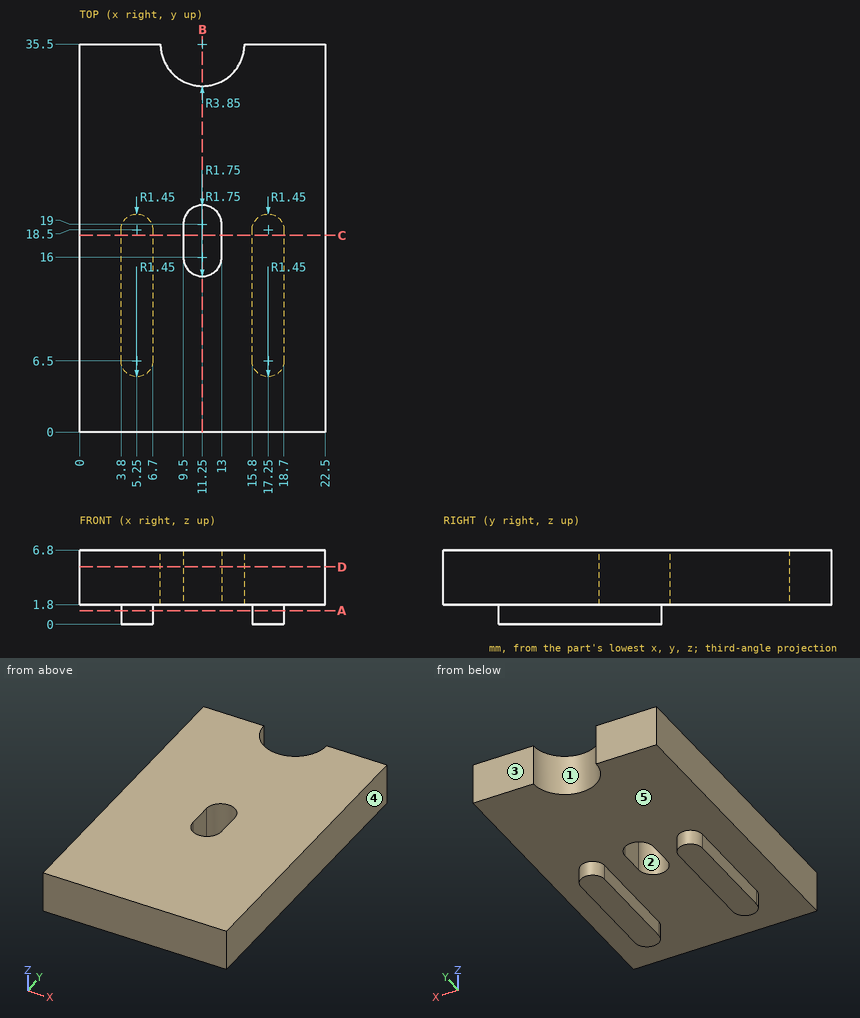
Can you work these out from the drawing? Everything is in mm from the part's minimum corner. A direction names the side the tool comes from. Round coordinates to 2 decimals unless told otherwise and drop trailing zeros. Loops run counter-clockwise (first coordinate to the right, second up) from the corner with the lowest first, then second, coordinate; pieces in that order, holes last. Notation, with made-up numbers: (21, 80.25) - (59, 80.25) arc R12 ccw to (59, 100.25) - close; hole circle Ø11 at (68, 62). An arc over 180 degrees is marked (long way). One line per question, with ' | ' between items. Start each with the question number.
Q1. I want a section at C-C (y = 18). Write out the boundary of the cut face in (x, z), then the cut area to 3 significant figures.
Q2. We'd pull the mould along X, two halves only. Please class the marked faces 3, 4 and 5: +X half, -X half, draft (parallel to the pull), parting line (faces both ways), or undercut.
Q3. For the marked faces 1 and 2, which set-ups out of +Z, -Z, +X, -X, +Y, -Y let a thin tool reach every point of the face, with its end or its side?
Q4. Please list where these lines run through material, in increasing order: line 1 (X direction, y = 16.5, z = 5); line 2 (X direction, y = 15.5, z = 0.5); line 3 (Z direction, x = 14.75, y = 27). Write a range as [from, to].
Q5. I want a section at B-B (x = 11.25). Write out the boundary of the cut face in (y, z).
Q6. I want a section at D-D (z = 5.25). Write out the boundary of the cut face in (x, y), then the cut area to 3 significant figures.
Q7. Will these pins go through, and if not, where does the flat tip stop? pin 1 (0.5 mm diameter, centred on y = 11, z = 1, fed in from +X); pin 2 (0.5 mm diameter, centred on y = 13, z = 1, fed in from -X).
Q8. I want a section at A-A (z = 1.25). Write out the boundary of the cut face in (x, y), then the cut area to 3 significant figures.
Response values:
1) outline: (0, 1.8) - (3.8, 1.8) - (3.8, 0) - (6.7, 0) - (6.7, 1.8) - (9.5, 1.8) - (9.5, 6.8) - (0, 6.8) - close; (13, 1.8) - (15.8, 1.8) - (15.8, 0) - (18.7, 0) - (18.7, 1.8) - (22.5, 1.8) - (22.5, 6.8) - (13, 6.8) - close | area: 105 mm²
2) face 3: draft | face 4: +X half | face 5: undercut
3) face 1: +Z, -Z, +Y | face 2: +Z, -Z
4) line 1: x = [0, 9.5], [13, 22.5] | line 2: x = [3.8, 6.7], [15.8, 18.7] | line 3: z = [1.8, 6.8]
5) outline: (0, 1.8) - (14.25, 1.8) - (14.25, 6.8) - (0, 6.8) - close; (20.75, 1.8) - (31.65, 1.8) - (31.65, 6.8) - (20.75, 6.8) - close
6) outline: (0, 0) - (22.5, 0) - (22.5, 35.5) - (15.1, 35.5) arc R3.85 cw to (7.4, 35.5) - (0, 35.5) - close; hole (9.5, 16) arc R1.75 ccw to (13, 16) - (13, 19) arc R1.75 ccw to (9.5, 19) - close | area: 755 mm²
7) pin 1: stops at x = 18.7 | pin 2: stops at x = 3.8
8) outline: (3.8, 6.5) arc R1.45 ccw to (6.7, 6.5) - (6.7, 18.5) arc R1.45 ccw to (3.8, 18.5) - close; (15.8, 6.5) arc R1.45 ccw to (18.7, 6.5) - (18.7, 18.5) arc R1.45 ccw to (15.8, 18.5) - close | area: 82.8 mm²
